Autodesk Inventor part; units mm, degrees
ref_plane "YZ Plane" through (0, 0, 0) normal (1, 0, 0) x (0, 1, 0)
ref_plane "XZ Plane" through (0, 0, 0) normal (0, 1, 0) x (-1, 0, 0)
ref_plane "XY Plane" through (0, 0, 0) normal (0, 0, 1) x (1, 0, 0)
sketch "Sketch1" plane through (0, 0, 0) normal (0, 0, 1) x (1, 0, 0)
  line L0 (0, 0) -> (-177.8, 0) construction
  line L1 (0, 69.85) -> (-177.8, 69.85)
  line L2 (-177.8, -69.85) -> (0, -69.85)
  arc A0 (0, -69.85) -> (0, 69.85) centre (0, 0) ccw
  arc A1 (-177.8, 69.85) -> (-177.8, -69.85) centre (-177.8, 0) ccw
  point P0 (-88.9, 0)
  dimension "d0" = 177.8
  dimension "d1" = 139.7
extrude "Extrusion1" add sketch "Sketch1" along normal blind 146.05
shell "Shell1" thickness 19.05 removed faces 1 at (-59.2667, -23.2833, 0)
sketch "Sketch2" plane through (-177.8, 69.85, 0) normal (0, 1, 0) x (1, 0, 0)
  line L0 (177.8, 0) -> (0, 0)
  line L1 (0, 0) -> (0, -146.05)
  line L2 (177.8, -146.05) -> (0, -146.05)
  line L3 (177.8, 0) -> (177.8, -146.05)
  line L4 (0, 0) -> (0, -146.05)
  line L5 (0, -73.025) -> (177.8, -73.025)
  line L6 (177.8, 0) -> (177.8, -127)
  line L7 (177.8, 0) -> (177.8, -146.05)
  line L8 (127, -73.025) -> (50.8, -73.025) construction
  line L9 (127, -53.975) -> (50.8, -53.975)
  line L10 (50.8, -92.075) -> (127, -92.075)
  arc A0 (127, -92.075) -> (127, -53.975) centre (127, -73.025) ccw
  arc A1 (50.8, -53.975) -> (50.8, -92.075) centre (50.8, -73.025) ccw
  point P0 (88.9, -73.025)
  dimension "d10" = 38.1
  dimension "d11" = 38.1
extrude "Extrusion2" cut sketch "Sketch2" against normal up to surface (19.05 mm away) contours A0 L10 A1 L5 | L5 A1 L9 A0
properties part number "Concrete case" material "GFRC"
Geometry: final body of the model. Coordinates: model frame, mm. A direction names the side the tool comes from. Round coordinates to 2 decimals unless told otherwise and drop trailing zeros. Write each loop counter-clockwise with the first axis right and the second up, starting at its lowest first coordinate (ties: lowest second). Pieces come first, ordered by that corner, then holes.
Item 1: Section query C-C (y = 0). Return loops of the section in (x, z), plus the area to 3 significant figures.
Item 2: Section query A-A (x = -58.5). Return loops of the section in (y, z) (3 decimals), plus the area to 3 significant figures.
Item 3: Section query B-B (z = 25.5). Return loops of the section in (x, y), plus the area to 3 significant figures.
Item 4: Material intervals for L1, parallel to Y at x = -158.5, z = 27; L2, parallel to X at y = -2, z = 66; L3, parallel to Z at x = -25, y = -13.5, sorted ascending.
Item 5: Mould query, pull axis X, two halves, no side actions, for faces 4 (the face through (-91, 1, 146.05)), 5 (the face through (-247.633, -1.536, 72.003)), 6 (the face through (50.788, 1.117, 62.611)). Classes: +X half, -X half, draft (parallel to the pull), parting line (faces both ways), or undercut.
Item 6: Section query D-D (z = 67). Return loops of the section in (x, y).
Item 7: Set-up query: faces 1 (the face through (-91, 1, 127)), 2 (the face through (69.833, 1.536, 72.003)), 3 (the face through (-88, 60, 53.975)). Return all of +Z, -Z, +X, -X, +Y, -Y with unobstructed straight access to the full face (end or side cutting, diameter ignored); none if empty.
Item 8: Pin query (flat end, axial travel): P1, Ø3, axis at y = -28.5, z = 95, coming from the +X side; P2, Ø1, axis at x = -215, z = 94, coming from the -Y side; P3, Ø1, axis at y = 49.5, z = 58.5, coming from the -X side. Return the tip coordinate at first contact, or that it passes through.
Completed:
1. outline: (-247.65, 0) - (-228.6, 0) - (-228.6, 127) - (50.8, 127) - (50.8, 0) - (69.85, 0) - (69.85, 146.05) - (-247.65, 146.05) - close
1. area: 10,900 mm2
2. outline: (-69.85, 0) - (-50.8, 0) - (-50.8, 127) - (50.8, 127) - (50.8, 92.075) - (69.85, 92.075) - (69.85, 146.05) - (-69.85, 146.05) - close; (50.8, 0) - (69.85, 0) - (69.85, 53.975) - (50.8, 53.975) - close
2. area: 6,770 mm2
3. outline: (-177.8, -69.85) - (0, -69.85) arc R69.85 ccw to (0, 69.85) - (-177.8, 69.85) arc R69.85 ccw to start; hole (-177.8, -50.8) - (0, -50.8) arc R50.8 ccw to (0, 50.8) - (-177.8, 50.8) arc R50.8 ccw to start
3. area: 14,000 mm2
4. L1: y = -69.85 to -50.8, 50.8 to 69.85
4. L2: x = -247.62 to -228.56, 50.76 to 69.82
4. L3: z = 127 to 146.05
5. face 4: draft
5. face 5: -X half
5. face 6: undercut
6. outline: (-177.8, -69.85) - (0, -69.85) arc R69.85 ccw to (0, 69.85) - (-32.73, 69.85) - (-32.73, 50.8) - (0, 50.8) arc R50.8 cw to (0, -50.8) - (-177.8, -50.8) arc R50.8 cw to (-177.8, 50.8) - (-145.07, 50.8) - (-145.07, 69.85) - (-177.8, 69.85) arc R69.85 ccw to start
7. face 1: -Z
7. face 2: +Z, -Z, +X
7. face 3: +Y
8. P1: stops at x = 64.42
8. P2: stops at y = -59.43
8. P3: stops at x = -227.58
